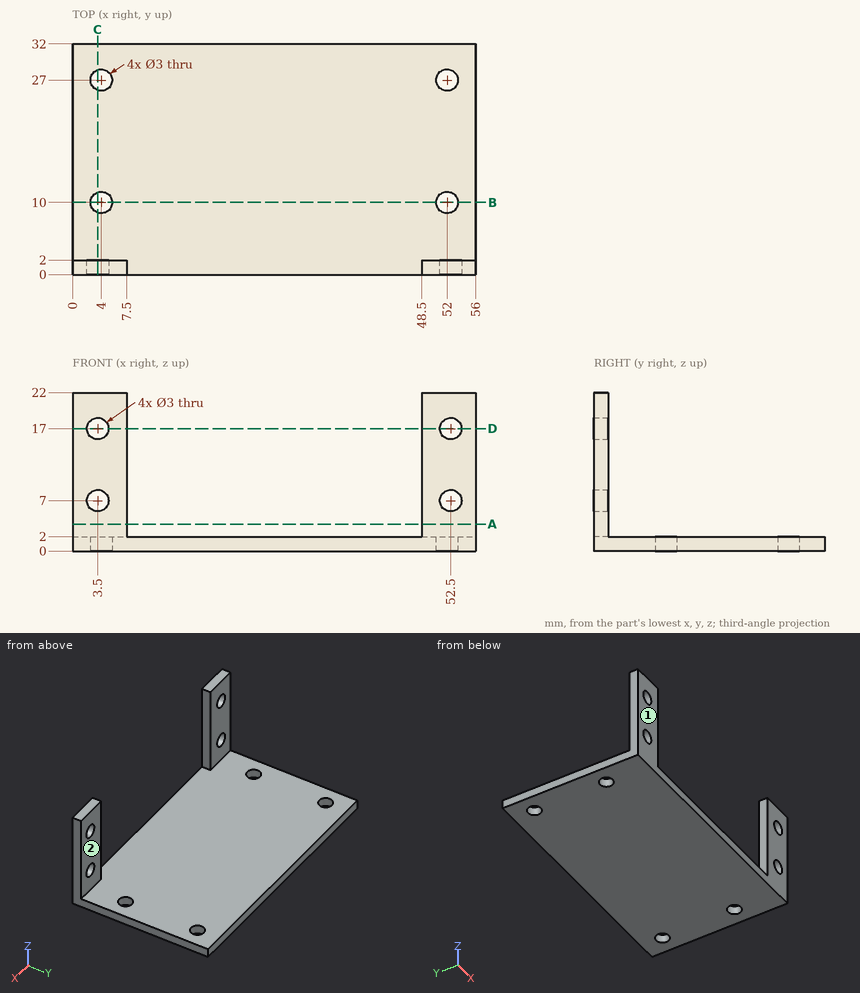
Answer from the drawing. Dimensions are ordinates in mm from the lowest x, y and z of the part. A direction names the side the tool comes from. Coordinates: 2 decimals unless noted, no trailing zeros. Write each loop counter-clockwise with the first axis right and the second up, starting at its lowest first coordinate (ties: lowest second). Pieces come first, ordered by that corner, then holes. Notation, with made-up numbers: (85, 63.25) -> (104, 63.25) arc R15 cw to (104, 89.25) -> close; hole circle Ø10 at (10.5, -8). An arc over 180 degrees is marked (long way). One line per question, with ' | ' between items.
1. Section A-A (z = 3.75) is taken. Determine the outline of the cut face in (x, y), and give its area (3 significant figures).
Verdict:
outline: (0, 0) -> (7.5, 0) -> (7.5, 2) -> (0, 2) -> close; (48.5, 0) -> (56, 0) -> (56, 2) -> (48.5, 2) -> close | area: 30.0 mm^2
2. Section C-C (x = 3.5) is taken. Determine the outline of the cut face in (y, z).
Verdict:
outline: (0, 0) -> (8.59, 0) -> (8.59, 2) -> (2, 2) -> (2, 5.5) -> (0, 5.5) -> close; (0, 8.5) -> (2, 8.5) -> (2, 15.5) -> (0, 15.5) -> close; (0, 18.5) -> (2, 18.5) -> (2, 22) -> (0, 22) -> close; (11.41, 0) -> (25.59, 0) -> (25.59, 2) -> (11.41, 2) -> close; (28.41, 0) -> (32, 0) -> (32, 2) -> (28.41, 2) -> close
3. Section B-B (y = 10) is taken. Determine the outline of the cut face in (x, z), and give its area (3 significant figures).
Verdict:
outline: (0, 0) -> (2.5, 0) -> (2.5, 2) -> (0, 2) -> close; (5.5, 0) -> (50.5, 0) -> (50.5, 2) -> (5.5, 2) -> close; (53.5, 0) -> (56, 0) -> (56, 2) -> (53.5, 2) -> close | area: 100 mm^2
4. Section D-D (z = 17) is taken. Determine the outline of the cut face in (x, y).
Verdict:
outline: (0, 0) -> (2, 0) -> (2, 2) -> (0, 2) -> close; (5, 0) -> (7.5, 0) -> (7.5, 2) -> (5, 2) -> close; (48.5, 0) -> (51, 0) -> (51, 2) -> (48.5, 2) -> close; (54, 0) -> (56, 0) -> (56, 2) -> (54, 2) -> close
5. Which of the six approach directions +Z, -Z, +X, -X, +Y, -Y give full straight-line access (tool end or side, diameter ignored) to the marked faces 1 and 2?
Verdict:
face 1: +Z, -Z, +X, -X, -Y | face 2: +Z, +X, -X, +Y
6. Straight lines are drawn through the part: line 1 (X direction, y = 1.6, z = 17); line 2 (Y direction, x = 4, z = 0.45); line 3 (Z direction, x = 49, y = 28). For each, find the intervals that lie inside material, in ascending order.
Verdict:
line 1: x = 0 to 2, 5 to 7.5, 48.5 to 51, 54 to 56 | line 2: y = 0 to 8.5, 11.5 to 25.5, 28.5 to 32 | line 3: z = 0 to 2
7. Given pin 1 Ø10 at (x, y) = (47.5, 22.5) entering from +Z; pin 2 Ø4 at (x, z) = (3.5, 7) entering from -Y; pin 3 Ø4 at (x, z) = (4.5, 13.5) entering from +Y, each flat-ended and moving along its own axis, determine where each tip first touches the part or whether it passes through.
Verdict:
pin 1: stops at z = 2 | pin 2: stops at y = 0 | pin 3: stops at y = 2
